Can you work these out from the model? Positions are in its coordinate system, mm. Face numbers are marked on the shaded views. Round coordinates to 2 decimals unless told otherwise and drop trailing zeros. Loops run counter-clockwise (first coordinate to the right, second up) from the corner with the lowest first, then second, coordinate; pieces in that order, holes last. Notation, with made-up numbers: (-25, -24.75) -> (1, -24.75) arc R12 ccw to (1, -13.75) -> close; hole circle Ø10 at (2.25, -27.75). An arc over 180 degrees is marked (long way). Write item = value, one per line.
from build123d import *

# Parameters (mm, degrees)
BOSS_EXTRUDE1_DEPTH      = 469.9
SKETCH2_W                = 10.16
SKETCH2_H                = 83.810703233
SKETCH2_H_2              = 111.159792755
SKETCH2_H_3              = 83.757510526
SKETCH2_H_4              = 83.784106879
SKETCH2_H_5              = 83.730914172
SKETCH2_H_6              = 83.704317819
SKETCH2_H_7              = 83.677721465
SKETCH2_H_8              = 83.651125112
SKETCH2_H_9              = 22.104476438
CUT_EXTRUDE1_DEPTH       = 10.16
SKETCH3_W                = 10.16
SKETCH3_H                = 55.879999965
SKETCH3_H_2              = 88.9
SKETCH3_H_3              = 109.22
CUT_EXTRUDE2_DEPTH       = 12.7
SKETCH4_W                = 81.316938584
SKETCH4_H                = 20.32
SKETCH4_W_2              = 81.316938585
CUT_EXTRUDE3_DEPTH       = 12.7
SKETCH5_W                = 89.916
SKETCH5_H                = 20.32
CUT_EXTRUDE4_DEPTH       = 12.7
SKETCH13_R               = 3.175
CUT_EXTRUDE8_DEPTH       = 2128.667464702
CUT_EXTRUDE9_DEPTH       = 2128.667464702
SKETCH20_R               = 4.7625
CUT_EXTRUDE10_DEPTH      = 2107.728843747
SKETCH24_R               = 3.175
CUT_EXTRUDE12_DEPTH      = 12.7
CUT_EXTRUDE13_DEPTH      = 2128.667464702
CUT_EXTRUDE13_DEPTH_BACK = 2128.667464702


with BuildPart() as part:
    # Sketch1 → Boss-Extrude1 (new body)
    with BuildSketch(Plane.XY):
        Polygon((-215.881789204, 2052.32), (-215.881789204, 1463.040000035), (-316.088635901, 20.32), (-317.499999939, 0), (-307.333509538, 0), (-205.715298803, 1463.040000035), (-205.715298803, 2072.64), (-215.881789204, 2072.64), align=None)
    extrude(amount=-BOSS_EXTRUDE1_DEPTH)

    # Sketch2 → Cut-Extrude1 (cut)
    with BuildSketch(Plane(origin=(-315.975651309, 21.946686571, 0), x_dir=(0, 0, 1), z_dir=(-0.9975965627192115, 0.06928995634877068, 0))):
        with Locations((-5.08, 247.132760087)):
            Rectangle(SKETCH2_W, SKETCH2_H)
        with Locations((-5.08, 55.684811679)):
            Rectangle(SKETCH2_W, SKETCH2_H_2)
        with Locations((-5.08, 602.706163733)):
            Rectangle(SKETCH2_W, SKETCH2_H_3)
        with Locations((-5.08, 424.91946191)):
            Rectangle(SKETCH2_W, SKETCH2_H_4)
        with Locations((-5.08, 780.492865556)):
            Rectangle(SKETCH2_W, SKETCH2_H_5)
        with Locations((-5.08, 958.27956738)):
            Rectangle(SKETCH2_W, SKETCH2_H_6)
        with Locations((-5.08, 1136.066269203)):
            Rectangle(SKETCH2_W, SKETCH2_H_7)
        with Locations((-5.08, 1313.852971026)):
            Rectangle(SKETCH2_W, SKETCH2_H_8)
        with Locations((-5.08, -10.947322918)):
            Rectangle(SKETCH2_W, SKETCH2_H_9)
        with Locations((-464.82, -10.947322918)):
            Rectangle(SKETCH2_W, SKETCH2_H_9)
        with Locations((-464.82, 55.684811679)):
            Rectangle(SKETCH2_W, SKETCH2_H_2)
        with Locations((-464.82, 247.132760087)):
            Rectangle(SKETCH2_W, SKETCH2_H)
        with Locations((-464.82, 424.91946191)):
            Rectangle(SKETCH2_W, SKETCH2_H_4)
        with Locations((-464.82, 602.706163733)):
            Rectangle(SKETCH2_W, SKETCH2_H_3)
        with Locations((-464.82, 780.492865556)):
            Rectangle(SKETCH2_W, SKETCH2_H_5)
        with Locations((-464.82, 958.27956738)):
            Rectangle(SKETCH2_W, SKETCH2_H_6)
        with Locations((-464.82, 1136.066269203)):
            Rectangle(SKETCH2_W, SKETCH2_H_7)
        with Locations((-464.82, 1313.852971026)):
            Rectangle(SKETCH2_W, SKETCH2_H_8)
    extrude(amount=-CUT_EXTRUDE1_DEPTH, mode=Mode.SUBTRACT)

    # Sketch3 → Cut-Extrude2 (cut)
    with BuildSketch(Plane.ZY.offset(215.881789204)):
        with Locations((-5.08, 1490.980000018)):
            Rectangle(SKETCH3_W, SKETCH3_H)
        with Locations((-5.08, 1652.27)):
            Rectangle(SKETCH3_W, SKETCH3_H_2)
        Polygon((-469.9, 1463.040000035), (-459.713026258, 1463.040000035), (-453.620872406, 1546.589538567), (-463.753970086, 1547.328410273), (-457.607940173, 1631.616820512), (-447.474842492, 1630.877948806), (-441.328812579, 1715.166359045), (-451.461910259, 1715.905230751), (-445.315880346, 1800.19364099), (-435.182782665, 1799.454769284), (-429.036752752, 1883.743179522), (-439.169850432, 1884.482051228), (-433.023820518, 1968.770461467), (-422.890722838, 1968.031589761), (-415.263026258, 2072.64), (-469.9, 2072.64), align=None)
        with Locations((-5.08, 1830.07)):
            Rectangle(SKETCH3_W, SKETCH3_H_2)
        with Locations((-5.08, 2018.03)):
            Rectangle(SKETCH3_W, SKETCH3_H_3)
    extrude(amount=-CUT_EXTRUDE2_DEPTH, mode=Mode.SUBTRACT)

    # Sketch4 → Cut-Extrude3 (cut)
    with BuildSketch(Plane.ZY.offset(215.881789204)):
        with Locations((-376.086223632, 2062.48)):
            Rectangle(SKETCH4_W, SKETCH4_H)
        with Locations((-213.452346463, 2062.48)):
            Rectangle(SKETCH4_W_2, SKETCH4_H)
        with Locations((-50.818469292, 2062.48)):
            Rectangle(SKETCH4_W_2, SKETCH4_H)
    extrude(amount=-CUT_EXTRUDE3_DEPTH, mode=Mode.SUBTRACT)

    # Sketch5 → Cut-Extrude4 (cut)
    with BuildSketch(Plane(origin=(-315.975651309, 21.946686571, 0), x_dir=(0, 0, 1), z_dir=(-0.9975965627192115, 0.06928995634877068, 0))):
        with Locations((-414.782, -11.839561137)):
            Rectangle(SKETCH5_W, SKETCH5_H)
        with Locations((-234.95, -11.839561137)):
            Rectangle(SKETCH5_W, SKETCH5_H)
        with Locations((-55.118, -11.839561137)):
            Rectangle(SKETCH5_W, SKETCH5_H)
    extrude(amount=-CUT_EXTRUDE4_DEPTH, mode=Mode.SUBTRACT)

    # Sketch13 → Cut-Extrude8 (cut, through all)
    with BuildSketch(Plane.ZY.offset(215.881789204)):
        with Locations(Location((-25.246459893, 1731.87, 0), (0, 0, 270))):
            Circle(SKETCH13_R)
        with Locations(Location((-70.408959893, 1755.42, 0), (0, 0, 270))):
            Circle(SKETCH13_R)
        with Locations(Location((-182.408959893, 1755.42, 0), (0, 0, 270))):
            Circle(SKETCH13_R)
        with Locations(Location((-25.246459893, 1918.97, 0), (0, 0, 270))):
            Circle(SKETCH13_R)
        with Locations(Location((-47.788959893, 1865.42, 0), (0, 0, 270))):
            Circle(SKETCH13_R)
        with Locations(Location((-182.408959893, 1910.42, 0), (0, 0, 270))):
            Circle(SKETCH13_R)
        with Locations(Location((-117.078959893, 1910.42, 0), (0, 0, 270))):
            Circle(SKETCH13_R)
        with Locations(Location((-70.408959893, 1895.42, 0), (0, 0, 270))):
            Circle(SKETCH13_R)
        with Locations(Location((-317.028959893, 1865.42, 0), (0, 0, 270))):
            Circle(SKETCH13_R)
        with Locations(Location((-294.408959893, 1755.42, 0), (0, 0, 270))):
            Circle(SKETCH13_R)
        with Locations(Location((-317.028959893, 1785.42, 0), (0, 0, 270))):
            Circle(SKETCH13_R)
        with Locations(Location((-339.571459893, 1731.87, 0), (0, 0, 270))):
            Circle(SKETCH13_R)
        with Locations(Location((-339.571459893, 1918.97, 0), (0, 0, 270))):
            Circle(SKETCH13_R)
    extrude(amount=-CUT_EXTRUDE8_DEPTH, mode=Mode.SUBTRACT)

    # Sketch17 → Cut-Extrude9 (cut, through all)
    with BuildSketch(Plane.ZY.offset(215.881789204)):
        Polygon((-91.602336227, 1471.504269383), (-81.702736369, 1473.789772095), (-94.643375784, 1529.841839519), (-104.542975642, 1527.556336807), align=None)
        Polygon((-130.424254473, 1639.660471655), (-117.483615058, 1583.608404231), (-107.584015199, 1585.893906943), (-120.524654614, 1641.945974367), align=None)
    extrude(amount=-CUT_EXTRUDE9_DEPTH, mode=Mode.SUBTRACT)

    # Sketch20 → Cut-Extrude10 (cut, through all)
    with BuildSketch(Plane(origin=(-315.975651309, 21.946686571, 0), x_dir=(0, 0, 1), z_dir=(-0.9975965627192116, 0.06928995634876853, 0))):
        with Locations(Location((-35.56, 347.287639338, 0), (0, 0, 270))):
            Circle(SKETCH20_R)
        with Locations(Location((-35.56, 302.837639338, 0), (0, 0, 270))):
            Circle(SKETCH20_R)
        Polygon((-120.929306778, 445.712379572), (-154.823537638, 399.698212032), (-162.492565561, 405.347250509), (-128.598334701, 451.361418049), align=None)
    extrude(amount=-CUT_EXTRUDE10_DEPTH, mode=Mode.SUBTRACT)

    # Sketch24 → Cut-Extrude12 (cut)
    with BuildSketch(Plane.ZY.offset(215.881789204)):
        with Locations(Location((-39.313746491, 1670.454214013, 0), (0, 0, 270))):
            Circle(SKETCH24_R)
    extrude(amount=-CUT_EXTRUDE12_DEPTH, mode=Mode.SUBTRACT)

    # Sketch26 → Cut-Extrude13 (cut, two sides: drawn at the far end of the back side and taken through both)
    with BuildSketch(Plane.ZY.offset(215.881789204).offset(-CUT_EXTRUDE13_DEPTH_BACK)):
        Polygon((-117.688081031, 385.528057798), (-109.500847052, 379.511801077), (-55.568463259, 452.553412636), (-63.755697238, 458.569669358), align=None)
        Polygon((-171.620464825, 312.486446238), (-225.552848619, 239.444834679), (-217.372552167, 233.433675887), (-163.440168374, 306.475287447), align=None)
        Polygon((-22.52887933, 606.973028774), (-44.10850301, 653.102617965), (-53.31924736, 648.814478552), (-31.73962368, 602.684889361), align=None)
        Polygon((-74.89887104, 694.944067742), (-65.68812669, 699.232207156), (-87.26775037, 745.361796346), (-96.478494721, 741.073656933), align=None)
        Polygon((-279.485232413, 166.403223119), (-333.417616206, 93.36161156), (-325.230382227, 87.345354838), (-271.297998434, 160.386966398), align=None)
    extrude(amount=CUT_EXTRUDE13_DEPTH + CUT_EXTRUDE13_DEPTH_BACK, mode=Mode.SUBTRACT)


solid = part.part
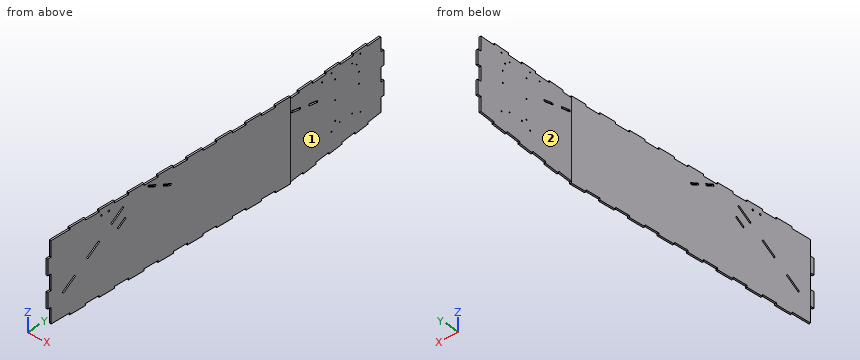
1. I need wall thicknesses on line 1 (Z direction, x = -211, y = 1755); line 2 (X direction, y = 1716.5, z = -360.5); line 3 (X direction, y = 162, z = -80.5). Which ranges of each line are inside material? Lowest first, please. Write a range as [from, to].
Entries:
line_1 = [-448.61, -297.56], [-291.26, -185.56], [-179.26, -73.56], [-67.26, 0]
line_2 = [-215.88, -205.72]
line_3 = [-306.25, -296.08]
2. Suppose I cut it at A-A, the plane y = 1335. List the corners of the cut face in (x, z) for me, and give its area (3 significant figures).
Entries:
outline = (-224.78, -459.74) -> (-214.61, -459.74) -> (-214.61, -10.16) -> (-224.78, -10.16) -> close
area = 4,570 mm²
3. I'm going to push flat-ended pins straight in: pin 1 (3 mm diameter, centred on x = -208.5, z = -6, fed in from +Y); pin 2 (8 mm diameter, centred on y = 212, z = -405, fed in from -X); pin 3 (8 mm diameter, centred on x = -212.5, z = -356.5, fed in from +Y); pin 4 (7.5 mm diameter, centred on y = 1731.87, z = -339.57, fed in from +X). Where does each tip first touch, or does it pass through?
Entries:
pin_1 = 1963.42
pin_2 = -303.05
pin_3 = 2052.32
pin_4 = -205.72
4. We'd pull the mould along X, two halves only. Please class the marked faces 1 and 2: released by +X, released by -X, zero draft, split by the parting line, or undercut.
Entries:
face_1 = released by +X
face_2 = released by -X
